Input: part model. Units: mm. Frame: model coordinates. Face numbers are marked on the shaded views. A direction names the side the tool comes from. Coordinates: 2 decimals unless noted, no trailing zeros. Loops run counter-clockwise (first coordinate to the right, second up) from the corner with the lowest first, then second, coordinate; pieces in that order, holes last.
(1) Line query: L1, parallel to X at y = 39.5, z = -2; L2, parallel to Z at x = -50, y = 15.75; L3, parallel to Y at x = -56, z = -8. Output: solid intervals per line, ascending.
(2) Contact query for flat-ended pins moving along their axis: P1, Ø11, axis at y = 3.5, z = 1, coming from the +X side; P2, Ø4, axis at x = -50, z = 0, coming from the -Y side; P3, Ø10, axis at x = -49, z = -2.5, coming from the -Y side. Output: stop coordinate, or through.
(3) Set-up query: the marked faces 1, 2 and 3. Return all of +Z, -Z, +X, -X, +Y, -Y with unobstructed straight access to the full face (end or side cutting, diameter ignored); none if empty.
(4) Section B-B, the plane z = 7. Return loops of the section in (x, y), then the cut area to 3 significant figures.
(5) Section A-A, the plane y = 46. Return loops of the section in (x, z), then the cut area to 3 significant figures.
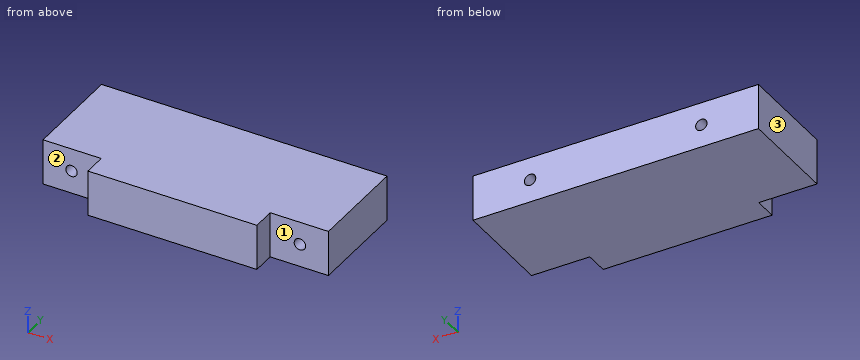
```python
from build123d import *

# Parameters (mm, degrees)
BOSS_EXTRUDE1_DEPTH   = 10
M6_TAPPED_HOLE1_D     = 5
M6_TAPPED_HOLE1_DEPTH = 15
M6_TAPPED_HOLE1_TIP   = 1.502151548
M6_TAPPED_HOLE2_D     = 5
M6_TAPPED_HOLE2_DEPTH = 15
M6_TAPPED_HOLE2_TIP   = 1.502151548


with BuildPart() as part:
    # Sketch1 → Boss-Extrude1 (new body, symmetric)
    with BuildSketch(Plane.XY):
        Polygon((-37, 0), (37, 0), (37, 10), (62.5, 10), (62.5, 54), (-62.5, 54), (-62.5, 10), (-37, 10), align=None)
    extrude(amount=BOSS_EXTRUDE1_DEPTH, both=True)

    # M6 Tapped Hole1
    with Locations(Plane(origin=(0, 10, 0), x_dir=(-1, 0, 0), z_dir=(0, -1, 0))):
        with Locations((50, 0), (-50, 0)):
            Hole(M6_TAPPED_HOLE1_D / 2, depth=M6_TAPPED_HOLE1_DEPTH)
            with Locations((0, 0, -(M6_TAPPED_HOLE1_DEPTH + M6_TAPPED_HOLE1_TIP / 2))):  # 118° drill point
                Cone(0, M6_TAPPED_HOLE1_D / 2, M6_TAPPED_HOLE1_TIP, mode=Mode.SUBTRACT)

    # M6 Tapped Hole2
    with Locations(Plane(origin=(0, 54, 0), x_dir=(1, 0, 0), z_dir=(0, 1, 0))):
        with Locations((-37.5, 0), (37.5, 0)):
            Hole(M6_TAPPED_HOLE2_D / 2, depth=M6_TAPPED_HOLE2_DEPTH)
            with Locations((0, 0, -(M6_TAPPED_HOLE2_DEPTH + M6_TAPPED_HOLE2_TIP / 2))):  # 118° drill point
                Cone(0, M6_TAPPED_HOLE2_D / 2, M6_TAPPED_HOLE2_TIP, mode=Mode.SUBTRACT)


solid = part.part
```
Report:
1. L1: x = -62.5 to -39, -36 to 36, 39 to 62.5
1. L2: z = -10 to -2.5, 2.5 to 10
1. L3: y = 10 to 54
2. P1: stops at x = 37
2. P2: stops at y = 25.3
2. P3: stops at y = 10
3. face 1: +Z, -Z, +X, -Y
3. face 2: +Z, -Z, -X, -Y
3. face 3: +Z, -Z, -X, +Y, -Y
4. outline: (-62.5, 10) - (-37, 10) - (-37, 0) - (37, 0) - (37, 10) - (62.5, 10) - (62.5, 54) - (-62.5, 54) - close
4. area: 6,240 mm2
5. outline: (-62.5, -10) - (62.5, -10) - (62.5, 10) - (-62.5, 10) - close; hole circle Ø5 at (-37.5, 0); hole circle Ø5 at (37.5, 0)
5. area: 2,460 mm2
